Part model, mm, in its own coordinate system. Face numbers are marked on the shaded views. A direction names the side the tool comes from. Give positions to 0.01 mm unless a question says otherwise; leave off trailing zeros. Write each loop counter-clockwise with the first axis right and the second up, starting at its lowest first coordinate (ties: lowest second). Pieces come first, ordered by that corner, then holes.
```python
from build123d import *

# Parameters (mm, degrees)
F0_R     = 30
F0_R_2   = 2.5
F0_R_3   = 16.1
F0_R_4   = 7.315
F1_DEPTH = 14.9
F2_R     = 3.2
F3_DEPTH = 14.6
F4_R     = 3.2


with BuildPart() as f1:
    # F0 (on Top) → F1 (new body)
    with BuildSketch(Plane.XY):
        Circle(F0_R)
        with Locations((0, -22.3)):
            Circle(F0_R_2, mode=Mode.SUBTRACT)
        with Locations((-22.3, 0)):
            Circle(F0_R_2, mode=Mode.SUBTRACT)
        Circle(F0_R_3, mode=Mode.SUBTRACT)
        with Locations((22.3, 0)):
            Circle(F0_R_2, mode=Mode.SUBTRACT)
        with Locations((0, 22.3)):
            Circle(F0_R_2, mode=Mode.SUBTRACT)
        Circle(F0_R_3)
        Circle(F0_R_4, mode=Mode.SUBTRACT)
    extrude(amount=-F1_DEPTH)

    # F2
    f2_edges = [f1.edges().sort_by_distance(p)[0] for p in [
        (-30, 0, 0),
    ]]
    fillet(f2_edges, radius=F2_R)

    # F0 (on Top) → F3 (join)
    with BuildSketch(Plane.XY):
        Circle(F0_R_3)
        Circle(F0_R_4, mode=Mode.SUBTRACT)
    extrude(amount=F3_DEPTH)

    # F4
    f4_edges = [f1.edges().sort_by_distance(p)[0] for p in [
        (-16.1, 0, 14.6),
    ]]
    fillet(f4_edges, radius=F4_R)


solid = f1.part
```
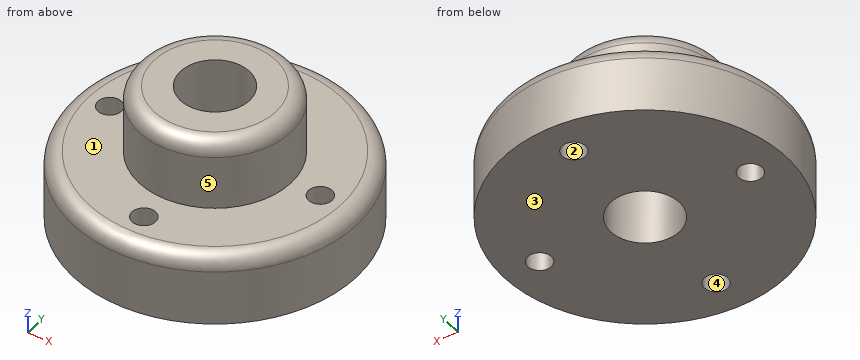
1) Wall check: L1, parallel to Y at x = 1, z = -3.5; L2, parallel to Z at x = 16.5, y = -2.5; L3, parallel to X at y = 21.5, z = -9. Give the ranges that are in metal, low to high.
Answers follow:
L1: y = -29.98 to -24.59, -20.01 to -7.25, 7.25 to 20.01, 24.59 to 29.98
L2: z = -14.9 to 0
L3: x = -20.92 to -2.37, 2.37 to 20.92
2) Pin check, flat tips, straight feed: pin 1 Ø4 at (x, z) = (-10, -5.5) entering from +Y; pin 2 Ø6.5 at (x, y) = (0, -22.3) entering from +Z; pin 3 Ø12 at (x, z) = (-19, -3.5) entering from -Y. Stop position of each tip, or through.
Answers follow:
pin 1: stops at y = 28.91
pin 2: stops at z = 0
pin 3: stops at y = -27.04
3) Saw through at D-D, the plane z = 1. Write the cut outline in (x, y) (3 decimals), then the cut area to 3 significant figures.
Answers follow:
outline: circle Ø32.2 at (0, 0); hole circle Ø14.63 at (0, 0)
area: 646 mm2
4) Two-plate mould, pull along X, no slides. Class the marked faces 3, 4 and 5: +X half, -X half, draft (parallel to the pull), parting line (faces both ways), or undercut.
Answers follow:
face 3: draft
face 4: undercut
face 5: parting line
5) 3-axis set-ups, long thin cutter, end or side, ignore diameter. For the marked faces 1 and 2: which of +Z, -Z, +X, -X, +Y, -Y reach the whole face in a straight line?
Answers follow:
face 1: +Z
face 2: +Z, -Z
6) Saw through at A-A, the plane y = 0. Write the cut outline in (x, z) (3 decimals), then the cut area to 3 significant figures.
Answers follow:
outline: (-30, -14.9) - (-24.8, -14.9) - (-24.8, 0) - (-26.8, 0) arc R3.2 ccw to (-30, -3.2) - close; (-19.8, -14.9) - (-7.315, -14.9) - (-7.315, 14.6) - (-12.9, 14.6) arc R3.2 ccw to (-16.1, 11.4) - (-16.1, 0) - (-19.8, 0) - close; (7.315, -14.9) - (19.8, -14.9) - (19.8, 0) - (16.1, 0) - (16.1, 11.4) arc R3.2 ccw to (12.9, 14.6) - (7.315, 14.6) - close; (24.8, -14.9) - (30, -14.9) - (30, -3.2) arc R3.2 ccw to (26.8, 0) - (24.8, 0) - close
area: 775 mm2
7) Saw through at C-C, the plane z = -4.5. Write the cut outline in (x, y) (3 decimals), then the cut area to 3 significant figures.
Answers follow:
outline: circle Ø60 at (0, 0); hole circle Ø5 at (-22.3, 0); hole circle Ø14.63 at (0, 0); hole circle Ø5 at (0, -22.3); hole circle Ø5 at (0, 22.3); hole circle Ø5 at (22.3, 0)
area: 2,580 mm2
